Can you work these out from the drawing? Everything is in mm from the part's minimum corner. Give positions to 0.01 mm unless a question says otherwise; leave off trailing zeros. Loops run counter-clockwise (first coordinate to the right, second up) from the corner with the lowest first, then second, coordinate; pieces in that order, holes last. Notation, with made-up numbers: (-22.5, 79.25) - (21.5, 79.25) arc R30 ccw to (21.5, 104.25) - close; hole circle Ø3 at (86.25, 51). An arc over 180 degrees is marked (long way). Write each question's results on one line, items separated by ' | '. Start each with the question number.
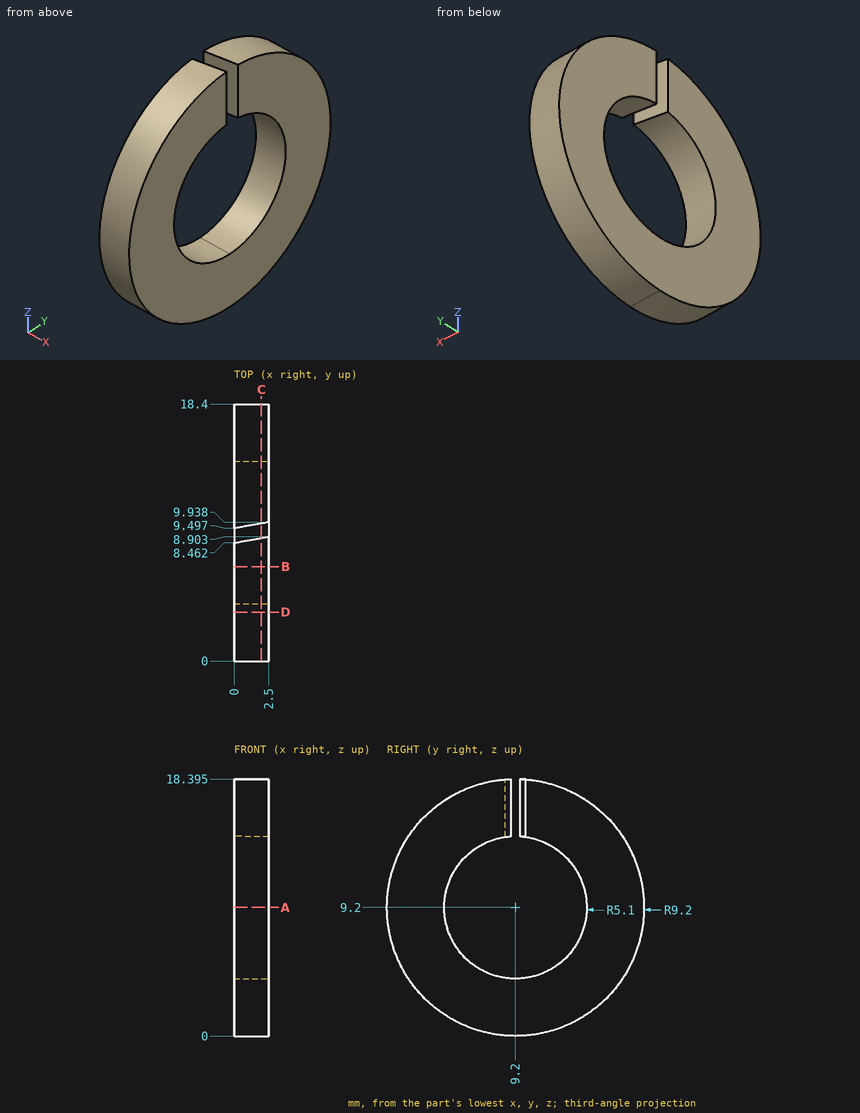
Q1. I want a section at C-C, the plane x = 1.95. List the corners of the cut face in (y, z) for me (1 decimal), then the cut area to 3 significant figures.
Q2. I need wall thicknesses on L1, parallel to Z at x = 1.15, y = 8; L2, parallel to Y at x = 1.05, z = 5.5 (1 decimal); L3, parallel to Y at x = 0.4, z = 10 (1 decimal). Which ranges of each line are inside material? Lowest first, please. Write a range as from..to.
Q3. I want a section at B-B, the plane y = 6.75. List the corners of the cut face in (x, z) for me.
Q4. I'm going to push flat-ended pins straight in: pin 1 Ø1.5 at (x, z) = (1.5, 9) entering from +Y; pin 2 Ø1.5 at (x, y) = (0.5, 6) entering from +Z; pin 3 Ø1.5 at (x, y) = (2, 3.5) entering from -Z (1 decimal). Where does each tip first touch, or does it pass through?
Q5. I want a section at D-D, the plane y = 3.5. List the corners of the cut face in (x, z) for me, then the cut area to 3 significant figures.
Q6. I want a section at A-A, the plane z = 9.2. List the corners of the cut face in (x, y) for me.
Conclusion:
1) outline: (8.8, 14.3) - (8.8, 18.4) arc R9.2 ccw (long way) to (9.8, 18.4) - (9.8, 14.3) arc R5.1 cw (long way) to start | area: 180 mm^2
2) L1: 0.08..4.24, 14.16..18.32 | L2: 0.8..5.7, 12.7..17.6 | L3: 0..4.2, 14.2..18.4
3) outline: (0, 0.33) - (2.5, 0.33) - (2.5, 4.73) - (0, 4.73) - close; (0, 13.67) - (2.5, 13.67) - (2.5, 18.07) - (0, 18.07) - close
4) pin 1: y = 18.4 | pin 2: z = 18.07 | pin 3: z = 1.4
5) outline: (0, 1.98) - (2.5, 1.98) - (2.5, 16.42) - (0, 16.42) - close | area: 36.1 mm^2
6) outline: (0, 0) - (2.5, 0) - (2.5, 4.1) - (0, 4.1) - close; (0, 14.3) - (2.5, 14.3) - (2.5, 18.4) - (0, 18.4) - close
